Part model, mm, in its own coordinate system. Face numbers are marked on the shaded views. Give positions to 0.01 mm unless a question says otherwise; leave off trailing zeros. Order: outer loops, then holes, each group sorted by start corner. A loop starts at its lowest first (then second) coordinate and runs counter-clockwise, first axis right, second up.
1. Probe line 1 (Y direction, x = -9, z = -22.5); line 2 (Y direction, x = -7, z = 78.5); line 3 (Y direction, x = -22.5, z = 78). List the from-to ranges inside material, lowest first.
2. Slice it at A-A on y = 99. List the corners of the cut face in (x, z), and give its area (3 significant figures).
3. Slice it at B-B on y = 61.5. List the corners of the cut face in (x, z), and give its area (3 significant figures).
4. Mould opens along Y. For the marked faces 1, 2 and 3 say: +Y half, -Y half, draft (parallel to the pull), parting line (faces both ways), or undercut.
5. Drop flat-ended pins along their axis: pin 1 Ø1.5 at (y, z) = (150.5, -31) entering from +X; pin 2 Ø5 at (x, z) = (-20.5, 71.5) entering from +Y. Give the stop position or say it passes through.
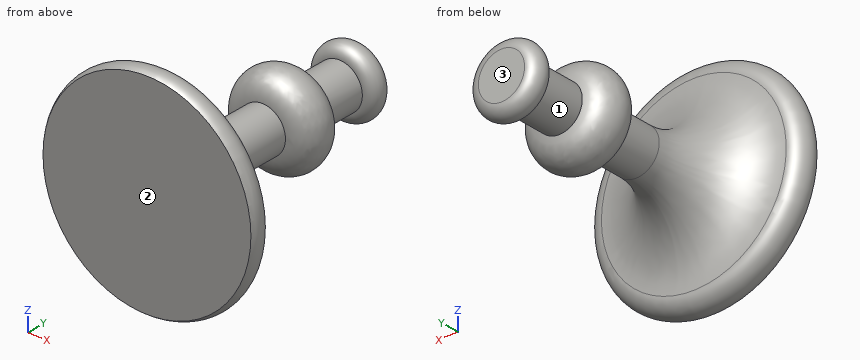
from build123d import *


with BuildPart() as part:
    # Sketch1 → Revolve1 (revolve)
    with BuildSketch(Plane.XY):
        with BuildLine():
            Line((0, 0), (0, 220))
            Line((0, 220), (20, 220))
            ThreePointArc((20, 220), (30, 210), (20, 200))
            Line((20, 200), (20, 160))
            ThreePointArc((20, 160), (40, 140), (20, 120))
            Line((20, 120), (20, 80.001263784))
            ThreePointArc((20, 80.001263784), (37.573593129, 37.574856913), (80, 20.001263784))
            ThreePointArc((80, 20.001263784), (91.180905073, 13.090889158), (90, 0))
            Line((90, 0), (0, 0))
        make_face()
    revolve(axis=Axis((0, 220, 0), (0, 1, 0)))


solid = part.part
Data:
1. line 1: y = 0 to 57.86, 120.45 to 159.55, 200.94 to 219.06
1. line 2: y = 0 to 20.01
1. line 3: y = 0 to 19.95
2. outline: circle Ø40 at (0, 0)
2. area: 1,260 mm2
3. outline: circle Ø45.85 at (0, 0)
3. area: 1,650 mm2
4. face 1: undercut
4. face 2: -Y half
4. face 3: +Y half
5. pin 1: stops at x = 21.6
5. pin 2: stops at y = 20.55
